```python
from build123d import *

# Parameters (mm, degrees)
SKETCH_1_R      = 7.5
EXTRUDE_1_DEPTH = 5


with BuildPart() as part:
    # Эскиз1 → Бобышка-Вытянуть1 (new body)
    with BuildSketch(Plane(origin=(0, 0, 0), x_dir=(1, 0, 0), z_dir=(0, 1, 0))):
        with BuildLine():
            Line((-17.116424198, -12.16667673), (-61.179242059, -56.229494591))
            Line((-61.179242059, -56.229494591), (-56.229494591, -61.179242059))
            Line((-56.229494591, -61.179242059), (-12.16667673, -17.116424198))
            ThreePointArc((-12.16667673, -17.116424198), (0, -21), (12.16667673, -17.116424198))
            Line((12.16667673, -17.116424198), (56.229494591, -61.179242059))
            Line((56.229494591, -61.179242059), (61.179242059, -56.229494591))
            Line((61.179242059, -56.229494591), (17.116424198, -12.16667673))
            ThreePointArc((17.116424198, -12.16667673), (21, 0), (17.116424198, 12.16667673))
            Line((17.116424198, 12.16667673), (61.179242059, 56.229494591))
            Line((61.179242059, 56.229494591), (56.229494591, 61.179242059))
            Line((56.229494591, 61.179242059), (12.16667673, 17.116424198))
            ThreePointArc((12.16667673, 17.116424198), (0, 21), (-12.16667673, 17.116424198))
            Line((-12.16667673, 17.116424198), (-56.229494591, 61.179242059))
            Line((-56.229494591, 61.179242059), (-61.179242059, 56.229494591))
            Line((-61.179242059, 56.229494591), (-17.116424198, 12.16667673))
            ThreePointArc((-17.116424198, 12.16667673), (-21, 0), (-17.116424198, -12.16667673))
        make_face()
        Circle(SKETCH_1_R, mode=Mode.SUBTRACT)
    extrude(amount=EXTRUDE_1_DEPTH)


solid = part.part
```
Verification items for the finished model (mm, model axes). A direction names the side the tool comes from. Coordinates: 2 decimals unless noted, no trailing zeros. Loops run counter-clockwise (first coordinate to the right, second up) from the corner with the lowest first, then second, coordinate; pieces in that order, holes last. Notation, with made-up numbers: (85.5, 17.25) -> (89.5, 17.25) arc R16 cw to (89.5, 47.25) -> close; hole circle Ø9 at (81.25, 33.25). An arc over 180 degrees is marked (long way). Put each result on its own line as item: value.
1. Mould release check, pull along Z, two halves, no side actions. Record for faces 1 (the face through (0, 0, -9)), 2 (the face through (39.46, 2.46, 34.51)), 3 (the face through (58.74, 2.46, -58.67)): pulls with the +Z half, pulls with the -Z half, needs draft (parallel to the pull), parting line crosses it, or undercut.
Result set:
face 1: needs draft
face 2: undercut
face 3: pulls with the -Z half
2. Thickness scan on line 1 (Z direction, x = 49, y = 3.6); line 2 (Z direction, x = -40, y = 3.1); line 3 (X direction, y = 3.8, z = -50.5). Record the ranges inside material, lowest first.
Result set:
line 1: z = -53.95 to -44.05, 44.05 to 53.95
line 2: z = -44.95 to -35.05, 35.05 to 44.95
line 3: x = -55.45 to -45.55, 45.55 to 55.45
3. Section check B-B, the plane y = 1.05. Record the boundary of the cut face in (x, z), then the cut area to 3 significant figures.
Result set:
outline: (-61.18, -56.23) -> (-56.23, -61.18) -> (-12.17, -17.12) arc R21 ccw to (12.17, -17.12) -> (56.23, -61.18) -> (61.18, -56.23) -> (17.12, -12.17) arc R21 ccw to (17.12, 12.17) -> (61.18, 56.23) -> (56.23, 61.18) -> (12.17, 17.12) arc R21 ccw to (-12.17, 17.12) -> (-56.23, 61.18) -> (-61.18, 56.23) -> (-17.12, 12.17) arc R21 ccw to (-17.12, -12.17) -> close; hole circle Ø15 at (0, 0)
area: 2,950 mm^2
4. Section check A-A, the plane x = 0. Record the boundary of the cut face in (y, z), then the cut area to 3 significant figures.
Result set:
outline: (0, -21) -> (5, -21) -> (5, -7.5) -> (0, -7.5) -> close; (0, 7.5) -> (5, 7.5) -> (5, 21) -> (0, 21) -> close
area: 135 mm^2
5. Tool access check on faces 4 (the face through (-34.51, 2.46, 39.46)), 5 (the face through (-38.84, 2.46, 33.89)), 6 (the face through (34.51, 2.46, -39.46)). Record the directions out of +Z, -Z, +X, -X, +Y, -Y that give a thin tool (end or side, any length) a straight path to the whole face; none if there is none.
Result set:
face 4: +Z, +Y, -Y
face 5: -X, +Y, -Y
face 6: -Z, +Y, -Y
6. Gauge pin test, flat ends, axial feed: P1, Ø3, axis at x = -4.5, y = 2.5, coming from the -Z side; P2, Ø6, axis at x = -28.5, z = 34.5, coming from the +Y side; P3, Ø3, axis at y = 3, z = 16.5, coming from the +X side; P4, Ø1, axis at y = 2, z = 47, coming from the -X side. Record the tip position at first contact, or that the pin passes through.
Result set:
P1: stops at z = -20.78
P2: stops at y = 5
P3: stops at x = 22.95
P4: stops at x = -52.45
7. Section check C-C, the plane z = 0. Record the boundary of the cut face in (x, y), then the cut area to 3 significant figures.
Result set:
outline: (-21, 0) -> (-7.5, 0) -> (-7.5, 5) -> (-21, 5) -> close; (7.5, 0) -> (21, 0) -> (21, 5) -> (7.5, 5) -> close
area: 135 mm^2
